The listing builds one solid part. Answer for the finished solid, in the listing's coordinates (mm). A direction names the side the tool comes from. Coordinates: 2 decimals unless noted, no trailing zeros. Order: outer loops, then holes, each group sorted by start corner. A loop starts at its lowest first (then second) coordinate and runs counter-clockwise, first axis right, second up. Notation, with made-up numbers: (60.25, 30.25) - (81.25, 30.25) arc R33 ccw to (81.25, 68.25) - close; hole circle Ø5 at (-37.75, 38). An arc over 180 degrees is marked (long way). Use one line per item in the form item = value. Start each with the question number.
Item 1: A tool of negligible diameter and unlimited length cuts with its end or side. For faces 1 (the flat face through (3, 1, 5)), 2 (the flat face through (0, -1.5, 12)), 3 (the cylindrical face through (3.233, -1.341, 2.465)), from which of +Z, -Z, +X, -X, +Y, -Y can it reach the whole face along a straight path? Write none if from no direction.
Item 2: Section A-A, the plane x = 0 is taken. Write down the section's boundary in (y, z), and give its area (3 significant figures).
Item 3: Section B-B, the plane y = 0 is taken. Write down the section's boundary in (x, z), and give its area (3 significant figures).
Item 4: Consider line 1 along Z through (x, y) = (-2, -2); line 2 along Z through (x, y) = (-1.75, -2.75); line 3 along X through (y, z) = (1.5, 12.75). Determine where each line is inside the solid, lowest interval first. Write a range as [from, to].
Item 5: Section C-C, the plane z = 10 is taken. Write down the section's boundary in (x, y), and give its area (3 significant figures).
Item 6: Section D-D, the plane y = 0.75 is taken. Write down the section's boundary in (x, z), and give its area (3 significant figures).
Item 7: Each of these flat-tipped pins is pushed along its axis until it touches: pin 1 Ø1 at (x, z) = (-0.5, 11.5) entering from -Y; pin 2 Ø1.5 at (x, z) = (1.5, 7) entering from -Y; pin 3 Ø0.8 at (x, y) = (1, -2) entering from +Z. Where does it stop, or does it pass through?
from build123d import *

# Parameters (mm, degrees)
SKETCH_R     = 3.5
PAD_DEPTH    = 5
SKETCH002_R  = 3
PAD001_DEPTH = 15
SKETCH003_W  = 6
SKETCH003_H  = 1.5
POCKET_DEPTH = 7


with BuildPart() as part:
    # Sketch → Pad (new body)
    with BuildSketch(Plane.XY):
        Circle(SKETCH_R)
    extrude(amount=PAD_DEPTH)

    # Sketch002 → Pad001 (join)
    with BuildSketch(Plane.XY):
        Circle(SKETCH002_R)
    extrude(amount=PAD001_DEPTH)

    # Sketch003 (on DatumPlane) → Pocket (cut)
    with BuildSketch(Plane.XY.offset(15)):
        with Locations((0, -2.25)):
            Rectangle(SKETCH003_W, SKETCH003_H)
    extrude(amount=-POCKET_DEPTH, mode=Mode.SUBTRACT)


solid = part.part
Response:
q1.face_1 = +Z
q1.face_2 = +Z, +X, -X, -Y
q1.face_3 = +Z, -Z
q2.outline = (-3.5, 0) - (3.5, 0) - (3.5, 5) - (3, 5) - (3, 15) - (-1.5, 15) - (-1.5, 8) - (-3, 8) - (-3, 5) - (-3.5, 5) - close
q2.area = 84.5 mm2
q3.outline = (-3.5, 0) - (3.5, 0) - (3.5, 5) - (3, 5) - (3, 15) - (-3, 15) - (-3, 5) - (-3.5, 5) - close
q3.area = 95.0 mm2
q4.line_1 = [0, 8]
q4.line_2 = [0, 5]
q4.line_3 = [-2.6, 2.6]
q5.outline = (-2.6, -1.5) - (2.6, -1.5) arc R3 ccw (long way) to start
q5.area = 22.7 mm2
q6.outline = (-3.42, 0) - (3.42, 0) - (3.42, 5) - (2.9, 5) - (2.9, 15) - (-2.9, 15) - (-2.9, 5) - (-3.42, 5) - close
q6.area = 92.3 mm2
q7.pin_1 = -1.5
q7.pin_2 = -2.9
q7.pin_3 = 8
